from build123d import *

# Parameters (mm, degrees)
SKETCH_1_R          = 2.1
SKETCH_1_W          = 15
SKETCH_1_H          = 15
EXTRUDE_1_DEPTH     = 5
CUT_EXTRUDE_1_DEPTH = 125.298028947
FILLET_1_R          = 3.005
FILLET_2_R          = 3.005


with BuildPart() as part:
    # ｽｹｯﾁ1 → ﾎﾞｽ - 押し出し1 (new body)
    # profile 1 of 3: a face of its own
    with BuildSketch(Plane.XY):
        Polygon((7.5, -7.5), (7.5, -22.5), (22.5, -7.5), (80, 50), (95, 50), (95, 65), (80, 80), (65, 80), (-7.5, 7.5), (7.5, 7.5), align=None)
        with Locations((72.5, 57.5)):
            Circle(SKETCH_1_R, mode=Mode.SUBTRACT)
        with Locations((87.5, 57.5)):
            Circle(SKETCH_1_R, mode=Mode.SUBTRACT)
        with Locations((72.5, 72.5)):
            Circle(SKETCH_1_R, mode=Mode.SUBTRACT)
    # profile 2 of 3: a face of its own
    with BuildSketch(Plane.XY):
        with Locations((0, -15)):
            Rectangle(SKETCH_1_W, SKETCH_1_H)
        with Locations((0, -15)):
            Circle(SKETCH_1_R, mode=Mode.SUBTRACT)
    # profile 3 of 3: a face of its own
    with BuildSketch(Plane.XY):
        Rectangle(SKETCH_1_W, SKETCH_1_H)
        Circle(SKETCH_1_R, mode=Mode.SUBTRACT)
    extrude(amount=EXTRUDE_1_DEPTH)

    # ｽｹｯﾁ2 → ｶｯﾄ - 押し出し1 (cut, through all)
    with BuildSketch(Plane.XY.offset(5)):
        Polygon((8.928932188, -14), (32.786796564, 9.857864376), (8.928932188, 9.857864376), align=None)
        Polygon((32.786796564, 16.857864376), (32.786796564, 40.715728753), (8.928932188, 16.857864376), align=None)
        Polygon((39.786796564, 16.857864376), (63.579405008, 40.65047282), (39.786796564, 40.707351623), align=None)
        Polygon((63.571067812, 47.650512753), (63.571067812, 71.5), (39.778459368, 47.707391556), align=None)
    extrude(amount=-CUT_EXTRUDE_1_DEPTH, mode=Mode.SUBTRACT)

    # ﾌｨﾚｯﾄ1
    fillet_1_edges = [part.edges().sort_by_distance(p)[0] for p in [
        (8.928932188, 9.857864376, 2.5),
        (32.786796564, 9.857864376, 2.5),
        (8.928932188, -14, 2.5),
        (32.786796564, 16.857864376, 2.5),
        (8.928932188, 16.857864376, 2.5),
        (32.786796564, 40.715728753, 2.5),
        (39.786796564, 40.707351623, 2.5),
        (63.579405008, 40.65047282, 2.5),
        (39.786796564, 16.857864376, 2.5),
        (63.571067812, 71.5, 2.5),
        (63.571067812, 47.650512753, 2.5),
        (39.778459368, 47.707391556, 2.5),
    ]]
    fillet(fillet_1_edges, radius=FILLET_1_R)

    # ﾌｨﾚｯﾄ2
    fillet_2_edges = [part.edges().sort_by_distance(p)[0] for p in [
        (-7.5, 7.5, 2.5),
        (65, 80, 2.5),
        (80, 80, 2.5),
        (95, 65, 2.5),
        (95, 50, 2.5),
        (80, 50, 2.5),
        (7.5, -22.5, 2.5),
        (-7.5, -22.5, 2.5),
    ]]
    fillet(fillet_2_edges, radius=FILLET_2_R)


solid = part.part
The listing builds one solid part. Answer for the finished solid, in the listing's coordinates (mm). A direction names the side the tool comes from. Coordinates: 2 decimals unless noted, no trailing zeros. Loops run counter-clockwise (first coordinate to the right, second up) from the corner with the lowest first, then second, coordinate; pieces in that order, holes last. Notation, with made-up numbers: M 73,48.25 L 114,48.25 A9 cw 114,64.25 Z; hole C -6,83.25 d2. An arc over 180 degrees is marked long. Answer in a Markdown table with one row per item.
1) Which of the six approach directions +Z, -Z, +X, -X, +Y, -Y give full straight-line access (tool end or side, diameter ignored) to faces 1 (the flat face through (36, 33, 5)), 2 (the cylindrical face through (28.327, 7.957, 2.465))?
Answers below:
| item | result |
|---|---|
| face 1 | +Z, +X, -X, +Y, -Y |
| face 2 | +Z, -Z |
2) Find section B-B (x = 0). Determine the outline of the cut face in (y, z).
Answers below:
| item | result |
|---|---|
| outline | M -22.5,0 L -17.1,0 L -17.1,5 L -22.5,5 Z; M -12.9,0 L -2.1,0 L -2.1,5 L -12.9,5 Z; M 2.1,0 L 15,0 L 15,5 L 2.1,5 Z |
3) Find the intervals of material crossed by probe 1 along Y at (x, z) = (22, 1.75); probe 2 along X at (y, z) = (30.5, 1.4); probe 3 along X at (y, z) = (28, 1.05), in increasing order.
Answers below:
| item | result |
|---|---|
| probe 1 | -8 to -0.93, 9.86 to 16.86, 29.93 to 37 |
| probe 2 | 15.5 to 22.57, 32.79 to 39.79, 53.43 to 60.5 |
| probe 3 | 13 to 20.07, 32.79 to 39.79, 50.93 to 58 |
4) Given pin 1 (1.5 mm diameter, centred on y = 29.5, z = 2.5, fed in from +X); pin 2 (2.5 mm diameter, centred on x = 0, y = 0, fed in from +Z); pin 3 (1.5 mm diameter, centred on y = 58, z = 1.5, fed in from -X); pin 4 (1.5 mm diameter, centred on x = 39, z = 1, fed in from +Y), each flat-ended and moving along its own axis, determine where each tip first touches the part or whether it passes through.
Answers below:
| item | result |
|---|---|
| pin 1 | x = 60.25 |
| pin 2 | through |
| pin 3 | x = 42.25 |
| pin 4 | y = 54.75 |
5) Find section C-C (y = -15). Determine the outline of the cut face in (x, z), then the cut area to 3 significant figures.
Answers below:
| item | result |
|---|---|
| outline | M -7.5,0 L -2.1,0 L -2.1,5 L -7.5,5 Z; M 2.1,0 L 15,0 L 15,5 L 2.1,5 Z |
| area | 91.5 mm^2 |
6) Find section D-D (y = 57.5). Determine the outline of the cut face in (x, z), then the cut area to 4 significant figures.
Answers below:
| item | result |
|---|---|
| outline | M 42.5,0 L 49.57,0 L 49.57,5 L 42.5,5 Z; M 63.57,0 L 70.4,0 L 70.4,5 L 63.57,5 Z; M 74.6,0 L 85.4,0 L 85.4,5 L 74.6,5 Z; M 89.6,0 L 95,0 L 95,5 L 89.6,5 Z |
| area | 150.5 mm^2 |
7) Find section A-A (x = 87.5). Determine the outline of the cut face in (y, z).
Answers below:
| item | result |
|---|---|
| outline | M 50,0 L 55.4,0 L 55.4,5 L 50,5 Z; M 59.6,0 L 72.5,0 L 72.5,5 L 59.6,5 Z |
8) Determine the mould class of faces 3 (the flat face through (-7.5, -7, 2)), 4 (the flat face through (73, 80, 2)), 5 (the flat face through (23, 16.858, 3)), 6 (the cylindrical face through (-6.64, -21.6, 2.54)) for opening direction Y: released by +Y, released by -Y, zero draft, split by the parting line, or undercut.
Answers below:
| item | result |
|---|---|
| face 3 | zero draft |
| face 4 | released by +Y |
| face 5 | undercut |
| face 6 | released by -Y |
